Model file for the job. Use its own axes, mm. Face numbers are marked on the shaded views. A direction names the side the tool comes from. Give positions to 0.01 mm unless a question says otherwise; leave off trailing zeros. Write each loop counter-clockwise with the first axis right and the second up, starting at its lowest first coordinate (ties: lowest second). Pieces come first, ordered by that corner, then holes.
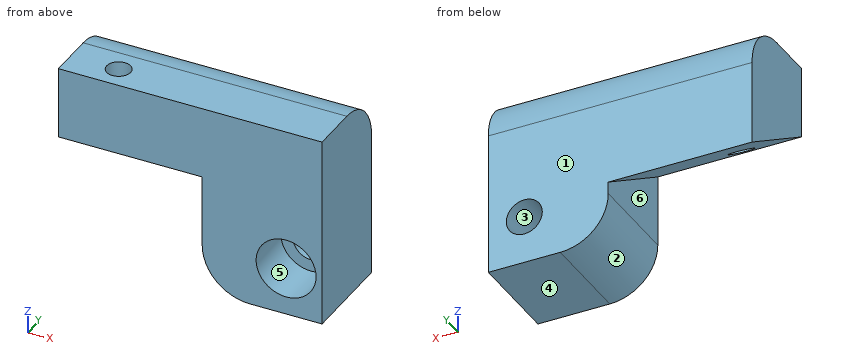
```python
from build123d import *

# Parameters (mm, degrees)
F0_R           = 15.875
F0_W           = 76.2
F0_H           = 69.85
F1_DEPTH       = 50.8
F2_R           = 25.4
F3_R           = 25.4
F5_SIZE2       = 31.743353
F5_SIZE        = 50.79999
F7_D           = 12.7
F8_D           = 19.05
F8_CBORE_D     = 31.75
F8_CBORE_DEPTH = 25.4


# Not quite as in the source:
# - a fillet or chamfer is up to 0.001 mm smaller than in the source, because OpenCascade refuses the exact size


with BuildPart() as f1:
    # F0 (on Front) → F1 (new body)
    with BuildSketch(Plane.XZ):
        Polygon((65.6778021347, 50.8), (2.1778021347, 50.8), (2.1778021347, -19.05), (2.1778021347, -50.8), (65.6778021347, -50.8), align=None)
        with Locations((46.6278021347, -25.4)):
            Circle(F0_R, mode=Mode.SUBTRACT)
        with Locations((46.6278021347, -25.4)):
            Circle(F0_R)
        with Locations((-35.9221978653, 15.875)):
            Rectangle(F0_W, F0_H)
    extrude(amount=F1_DEPTH)

    # F2
    f2_edges = [f1.edges().sort_by_distance(p)[0] for p in [
        (2.177802, -25.4, -50.8),
    ]]
    fillet(f2_edges, radius=F2_R)

    # F3
    f3_edges = [f1.edges().sort_by_distance(p)[0] for p in [
        (-4.172198, 0, 50.8),
    ]]
    fillet(f3_edges, radius=F3_R)

    # F5 (size 50.8 and 31.743363077 in the source; OpenCascade refuses exactly that, so slightly less here)
    f5_edges = [f1.edges().sort_by_distance(p)[0] for p in [
        (-35.922198, -50.8, -19.05),
    ]]
    f5_side = f1.faces().sort_by_distance((-35.922198, -25.4, -19.05))[0]
    chamfer(f5_edges, length=F5_SIZE, length2=F5_SIZE2, reference=f5_side)

    # F7 (through all)
    with Locations(Plane.XY.offset(50.8)):
        with Locations((-48.6221978653, -38.1)):
            Hole(F7_D / 2)

    # F8 (through all)
    with Locations(Plane.XZ.offset(50.8)):
        with Locations((46.6278021347, -25.4)):
            CounterBoreHole(F8_D / 2, F8_CBORE_D / 2, F8_CBORE_DEPTH)


solid = f1.part
```
1. Slice it at D-D, the plane z = 31. Write the cut outline in (x, y).
Calculated:
outline: (-74.02, -50.8) - (65.68, -50.8) - (65.68, -0.63) - (-74.02, -0.63) - close; hole circle Ø12.7 at (-48.62, -38.1)
2. Probe probe 1 along X at (y, z) = (-38, 11); probe 2 along Z at (x, y) = (46.5, -41); probe 3 along X at (y, z) = (-44, -25). List the from-to ranges inside material, lowest first.
Calculated:
probe 1: x = -74.02 to -54.97, -42.27 to 65.68
probe 2: z = -50.8 to -41.27, -9.53 to 50.8
probe 3: x = 2.18 to 30.76, 62.5 to 65.68
3. Slice it at C-C, the plane y = -47.5. Write the cut outline in (x, z) (3 decimals), and give its area (3 significant figures).
Calculated:
outline: (-74.022, 10.631) - (2.178, 10.631) - (2.178, -25.4) arc R25.4 ccw to (27.578, -50.8) - (65.678, -50.8) - (65.678, 50.8) - (-74.022, 50.8) - close; hole circle Ø31.75 at (46.628, -25.4)
area: 8,580 mm2
4. Slice it at B-B, the plane x = 54. Write the cut outline in (y, z), and give its area (3 significant figures).
Calculated:
outline: (-50.8, -50.8) - (0, -50.8) - (0, -31.43) - (-25.4, -31.43) - (-25.4, -39.46) - (-50.8, -39.46) - close; (-50.8, -11.34) - (-25.4, -11.34) - (-25.4, -19.37) - (0, -19.37) - (0, 25.4) arc R25.4 ccw to (-25.4, 50.8) - (-50.8, 50.8) - close
area: 4,000 mm2
5. Pull direction Z, two halves, no side cores. Call the marked faces 1, 2 and 3: +Z half, -Z half, draft (parallel to the pull), parting line (faces both ways), or undercut.
Calculated:
face 1: draft
face 2: -Z half
face 3: undercut
6. Slice it at A-A, the plane y = -40. Write the cut outline in (x, z) (3 decimals), and give its area (3 significant figures).
Calculated:
outline: (-74.022, 5.945) - (-54.681, 5.945) - (-54.681, 50.8) - (-74.022, 50.8) - close; (-42.563, 5.945) - (2.178, 5.945) - (2.178, -25.4) arc R25.4 ccw to (27.578, -50.8) - (65.678, -50.8) - (65.678, 50.8) - (-42.563, 50.8) - close; hole circle Ø31.75 at (46.628, -25.4)
area: 8,400 mm2
7. Pin check, flat tips, straight feed: P1, Ø1, axis at x = 41.5, z = 39.5, coming from the +Y side; P2, Ø1.5, axis at x = 32, y = -6.5, coming from the +Z side; P3, Ø11.5, axis at x = 46.63, z = -25.4, coming from the +Y side; P4, Ø1, axis at x = 25.5, y = -9.5, coming from the +Z side. Stop position of each tip, or through.
Calculated:
P1: stops at y = -3.95
P2: stops at z = 43.17
P3: passes through
P4: stops at z = 45.6
8. Which spindle directions (+Z, -Z, +X, -X, +Y, -Y) get a long thin tool onto all of the face, cutting with end or side? Do the marked faces 4, 5 and 6. Say none if no direction does.
Calculated:
face 4: -Z, +X, -X, +Y, -Y
face 5: -Y
face 6: -Z, -X, -Y
